from build123d import *
from OCP.BRepFilletAPI import BRepFilletAPI_MakeChamfer

# Parameters (mm, degrees)
SKETCH_1_R          = 10
EXTRUDE_1_DEPTH     = 24
SKETCH_4_R          = 16.025
CUT_EXTRUDE_3_DEPTH = 9
SKETCH_5_W          = 48
SKETCH_5_H          = 3
EXTRUDE_2_DEPTH     = 25
CHAMFER_1_SIZE      = 5
CHAMFER_1_SIZE2     = 8.660254038
SKETCH_7_R          = 1.6
CUT_EXTRUDE_4_DEPTH = 76.00666637
FILLET_1_R          = 20
FILLET_2_R          = 5


with BuildPart() as part:
    # 草图1 → 凸台-拉伸1 (new, symmetric)
    with BuildSketch(Plane.XY):
        Polygon((-20, -35), (-20, 0), (-20, 20), (20, 20), (20, 0), (20, -35), align=None)
        Circle(SKETCH_1_R, mode=Mode.SUBTRACT)
    extrude(amount=EXTRUDE_1_DEPTH, both=True)

    # 草图4 → 切除-拉伸3 (cut)
    with BuildSketch(Plane(origin=(0, 0, -24), x_dir=(-1, 0, 0), z_dir=(0, 0, -1))):
        Circle(SKETCH_4_R)
    cut_extrude_3 = extrude(amount=-CUT_EXTRUDE_3_DEPTH, mode=Mode.SUBTRACT)

    # 镜向1: 切除-拉伸3 across plane
    add(cut_extrude_3.mirror(Plane.XY), mode=Mode.SUBTRACT)

    # 草图5 → 凸台-拉伸2 (add)
    with BuildSketch(Plane(origin=(20, 0, 0), x_dir=(0, 0, -1), z_dir=(1, 0, 0))):
        with Locations((0, -33.5)):
            Rectangle(SKETCH_5_W, SKETCH_5_H)
    extrude_2 = extrude(amount=EXTRUDE_2_DEPTH)

    # 镜向2: 凸台-拉伸2 across plane
    add(extrude_2.mirror(Plane.ZY))

    # 倒角1: one chamfer whose edges measure the first distance from different faces: ONE call of the kernel's chamfer builder (chamfer() names one face for all edges)
    chamfer_1_edges_1 = [part.edges().sort_by_distance(p)[0] for p in [
        (20, -32, 0),
    ]]
    chamfer_1_side_1 = [part.faces().sort_by_distance(p)[0] for p in [
        (32.5, -32, 0),
    ]]
    chamfer_1_edges_2 = [part.edges().sort_by_distance(p)[0] for p in [
        (-20, -32, 0),
    ]]
    chamfer_1_side_2 = [part.faces().sort_by_distance(p)[0] for p in [
        (-32.5, -32, 0),
    ]]
    chamfer_1 = BRepFilletAPI_MakeChamfer(part.part.solid().wrapped)
    for e in chamfer_1_edges_1:
        chamfer_1.Add(CHAMFER_1_SIZE, CHAMFER_1_SIZE2, e.wrapped, chamfer_1_side_1[0].wrapped)  # the first distance lies on this face
    for e in chamfer_1_edges_2:
        chamfer_1.Add(CHAMFER_1_SIZE, CHAMFER_1_SIZE2, e.wrapped, chamfer_1_side_2[0].wrapped)  # the first distance lies on this face
    add(Compound.cast(chamfer_1.Shape()), mode=Mode.REPLACE)

    # 草图7 → 切除-拉伸4 (cut, through all)
    with BuildSketch(Plane.XZ.offset(35)):
        with Locations(Location((37.5, 14, 0), (0, 0, 270))):
            Circle(SKETCH_7_R)
        with Locations(Location((37.5, -14, 0), (0, 0, 270))):
            Circle(SKETCH_7_R)
        with Locations(Location((-37.5, 14, 0), (0, 0, 90))):
            Circle(SKETCH_7_R)
        with Locations(Location((-37.5, -14, 0), (0, 0, 90))):
            Circle(SKETCH_7_R)
    extrude(amount=-CUT_EXTRUDE_4_DEPTH, mode=Mode.SUBTRACT)

    # 圆角1
    fillet_1_edges = [part.edges().sort_by_distance(p)[0] for p in [
        (20, 20, 0),
        (-20, 20, 0),
    ]]
    fillet(fillet_1_edges, radius=FILLET_1_R - 0.0001)  # a hair under: the kernel refuses the full size

    # 圆角2
    fillet_2_edges = [part.edges().sort_by_distance(p)[0] for p in [
        (45, -33.5, 24),
        (45, -33.5, -24),
        (-45, -33.5, 24),
        (-45, -33.5, -24),
    ]]
    fillet(fillet_2_edges, radius=FILLET_2_R)


solid = part.part
CAD build for the part. Positions are in the model's coordinates, mm. A direction names the side the tool comes from. Round coordinates to 2 decimals unless told otherwise and drop trailing zeros. Write each loop counter-clockwise with the first axis right and the second up, starting at its lowest first coordinate (ties: lowest second). Pieces come first, ordered by that corner, then holes.
(1) Probe line 1 along X through (y, z) = (-34, 14); line 2 along Y through (x, z) = (0, -18.25) (3 decimals); line 3 along Y through (x, z) = (29, -9). List the from-to ranges inside material, lowest first.
(2) 3-axis set-ups, long thin cutter, end or side, ignore diameter. For faces 1 (the face through (12.72, -9.75, -19.56)), 2 (the face through (12.72, -9.75, 19.56)), 3 (the face through (20, -12, 0)): which of +Z, -Z, +X, -X, +Y, -Y reach the whole face in a straight line?
(3) Drop flat-ended pins along their axis: P1, Ø1.5, axis at x = 24.5, y = -29.5, coming from the -Z side; P2, Ø12, axis at y = -6.5, z = -7, coming from the +X side; P3, Ø10, axis at x = 34.5, z = 6.5, coming from the +Y side; P4, Ø18.5, axis at y = -16.5, z = -2.5, coming from the +X side. Give the stop position or say it passes through.
(4) Slice it at B-B, the plane x = -37.5. Write the cut outline in (y, z), and give its area (3 significant figures).
(5) Slice it at A-A, the plane z = -14. Count the separate pieces of the cut face and the enclosed holes in it, and give its area (3 significant figures).
(6) Slice it at D-D, the plane x = 2.5. Write the cut outline in (y, z).
(7) Mould opens along X. For faces 4 (the face through (22.465, -27.609, 0.336)), 5 (the face through (-45, -33, 0)), 6 (the face through (-35, -32, 0)), 7 (the face through (-10.5, 0.2, 15)) say: pulls with the +X half, pulls with the -X half, needs draft (parallel to the pull), parting line crosses it, or undercut.
From the geometry:
1. line 1: x = -45 to -39.1, -35.9 to 35.9, 39.1 to 45
1. line 2: y = -35 to -16.025, 16.025 to 20
1. line 3: y = -35 to -32
2. face 1: -Z
2. face 2: +Z
2. face 3: +Z, -Z, +X, +Y
3. P1: passes through
3. P2: stops at x = 20
3. P3: stops at y = -32
3. P4: stops at x = 21.39
4. outline: (-35, -24) - (-32, -24) - (-32, -15.6) - (-35, -15.6) - close; (-35, -12.4) - (-32, -12.4) - (-32, 12.4) - (-35, 12.4) - close; (-35, 15.6) - (-32, 15.6) - (-32, 24) - (-35, 24) - close
4. area: 125 mm2
5. separate pieces: 3
5. enclosed holes: 1
5. area: 1,890 mm2
6. outline: (-35, -24) - (-15.83, -24) - (-15.83, -15) - (-9.68, -15) - (-9.68, 15) - (-15.83, 15) - (-15.83, 24) - (-35, 24) - close; (9.68, -15) - (15.83, -15) - (15.83, -24) - (19.84, -24) - (19.84, 24) - (15.83, 24) - (15.83, 15) - (9.68, 15) - close
7. face 4: pulls with the +X half
7. face 5: pulls with the -X half
7. face 6: needs draft
7. face 7: undercut
